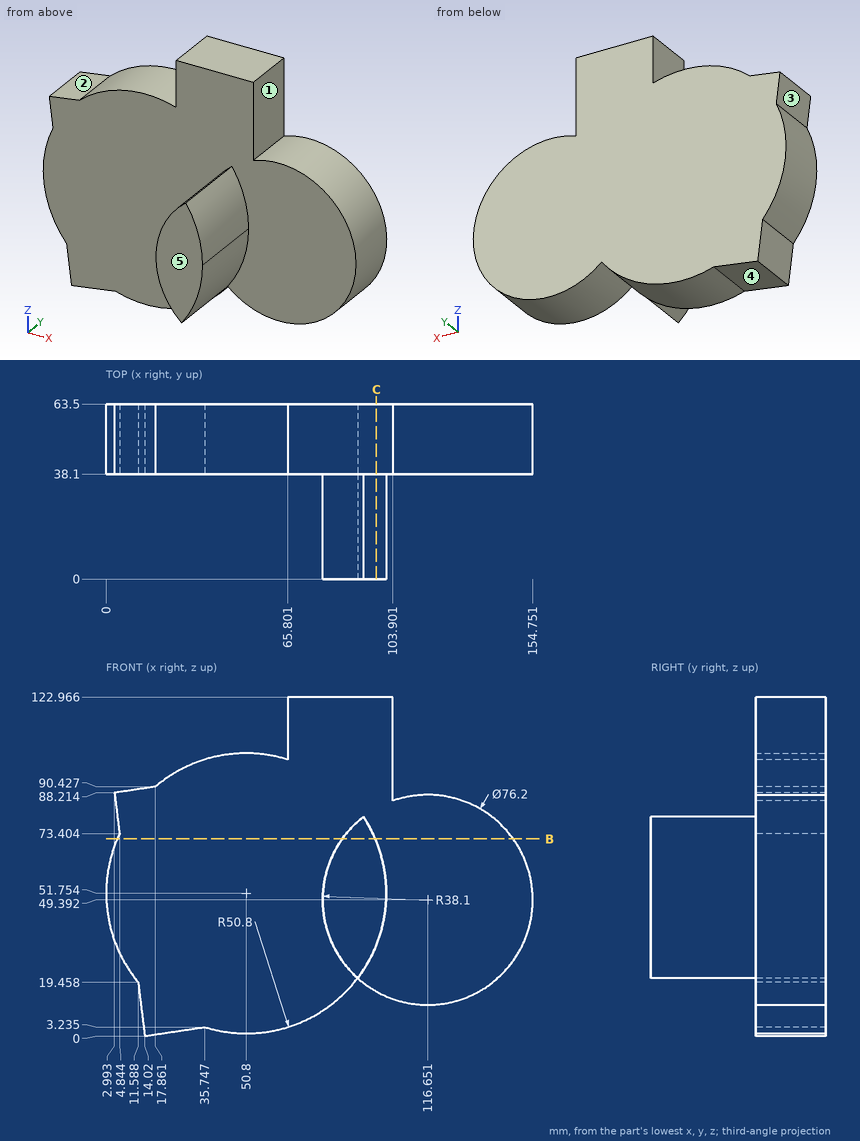
Part print with two shaded views. Sizes in mm from the minimum x, y, z corner. A direction names the side the tool comes from. Round coordinates to 2 decimals unless told otherwise and drop trailing zeros. Write each loop counter-clockwise with the first axis right and the second up, starting at its lowest first coordinate (ties: lowest second). Pieces come first, ordered by that corner, then holes. Notation, with made-up numbers: M -23,59.5 L 36,59.5 A22 ccw 36,78.5 Z; hole C 5,-24.75 d3. An arc over 180 degrees is marked long. Put each result on its own line as item: value. Start each with the question number.
1) Saw through at C-C, the plane x = 98. Write the cut outline in (y, z) (1 decimal), and give its area (3 significant figures).
2) Pull direction Z, two halves, no side cores. Call the marked faces 1, 2 and 3: pulls with the +Z half, pulls with the -Z half, needs draft (parallel to the pull), parting line crosses it, or undercut.
3) Drill centre lines: probe 1 along Y at (x, z) = (44.5, 78.5); probe 2 along X at (y, z) = (43, 23); probe 3 along Z at (x, y) = (108, 40). Where is each one in solid material? Low to high. Write a range as [from, to].
4) 3-axis set-ups, long thin cutter, end or side, ignore diameter. For the marked faces 4 and 5: which of +Z, -Z, +X, -X, +Y, -Y reach the whole face in a straight line?
5) Saw through at B-B, the plane z = 71.5. Write the cut outline in (x, y) (1 decimal).
6) Pin check, flat tips, straight feed: pin 1 Ø3 at (x, z) = (16, 90.5) entering from +Y; pin 2 Ø5 at (y, z) = (22, 72.5) entering from +X; pin 3 Ø12.5 at (y, z) = (52, 109.5) entering from +X; pin 4 Ø10 at (x, y) = (89.5, 28) entering from -Z. Stop position of each tip, or through.
Resolved:
1. outline: M 0,33 L 38.1,33 L 38.1,16.2 L 63.5,16.2 L 63.5,123 L 38.1,123 L 38.1,70.5 L 0,70.5 Z
1. area: 4,140 mm²
2. face 1: needs draft
2. face 2: pulls with the +Z half
2. face 3: undercut
3. probe 1: [38.1, 63.5]
3. probe 2: [8.92, 144.13]
3. probe 3: [12.29, 86.5]
4. face 4: -Z, +Y, -Y
4. face 5: +Z, -Z, +X, -X, -Y
5. outline: M 4,38.1 L 85.6,38.1 L 85.6,0 L 97.6,0 L 97.6,38.1 L 147.7,38.1 L 147.7,63.5 L 4,63.5 Z
6. pin 1: y = 63.5
6. pin 2: x = 98.21
6. pin 3: x = 103.9
6. pin 4: z = 21.01
